For this review, take the finished solid that the model builds, in its own axes (mm). A direction names the side the tool comes from. Give positions to 0.01 mm unless a question says otherwise; leave off trailing zeros. Write each loop counter-clockwise with the first axis right and the second up, starting at its lowest first coordinate (ties: lowest second). Pieces come first, ordered by that corner, then holes. Notation, with made-up numbers: (56, 16) -> (81, 16) arc R30 cw to (81, 54) -> close; hole circle Ø3 at (-32, 41). An arc over 180 degrees is marked (long way). Answer as CSV lines item,"result".
```python
from build123d import *

# Parameters (mm, degrees)
SKETCH1_R           = 1.5
BOSS_EXTRUDE1_DEPTH = 3


with BuildPart() as part:
    # Sketch1 → Boss-Extrude1 (new body)
    with BuildSketch(Plane.XY):
        with BuildLine():
            ThreePointArc((-0.08, 4), (-0.080376511, 3.999992452), (-0.080753021, 3.999984869))
            ThreePointArc((-0.080753021, 3.999984869), (0.560266414, 4.536513248), (1.110799577, 5.165545722))
            Line((1.110799577, 5.165545722), (0.873535849, 5.738351032))
            ThreePointArc((0.873535849, 5.738351032), (-0.292204471, 5.779997685), (-1.43969018, 5.570327744))
            ThreePointArc((-1.43969018, 5.570327744), (-1.699752868, 6.045), (-1.980799756, 6.507557022))
            ThreePointArc((-1.980799756, 6.507557022), (-1.225477407, 7.396473826), (-0.678674306, 8.426857884))
            Line((-0.678674306, 8.426857884), (-1.056106392, 8.918736955))
            ThreePointArc((-1.056106392, 8.918736955), (-2.192904021, 8.657248736), (-3.247023529, 8.15773197))
            ThreePointArc((-3.247023529, 8.15773197), (-3.621079015, 8.548920985), (-4.01226803, 8.922976471))
            ThreePointArc((-4.01226803, 8.922976471), (-3.512751264, 9.977095979), (-3.251263045, 11.113893608))
            Line((-3.251263045, 11.113893608), (-3.743142116, 11.491325694))
            ThreePointArc((-3.743142116, 11.491325694), (-4.773526174, 10.944522593), (-5.662442978, 10.189200244))
            ThreePointArc((-5.662442978, 10.189200244), (-6.125, 10.470247132), (-6.599672256, 10.73030982))
            ThreePointArc((-6.599672256, 10.73030982), (-6.390002315, 11.877795529), (-6.431648968, 13.043535849))
            Line((-6.431648968, 13.043535849), (-7.004454278, 13.280799577))
            ThreePointArc((-7.004454278, 13.280799577), (-7.858205794, 12.485945322), (-8.521341684, 11.526291359))
            ThreePointArc((-8.521341684, 11.526291359), (-9.040877745, 11.67804324), (-9.566685112, 11.806390286))
            ThreePointArc((-9.566685112, 11.806390286), (-9.661150657, 12.969042942), (-10.003094031, 14.084282677))
            Line((-10.003094031, 14.084282677), (-10.617789845, 14.165208916))
            ThreePointArc((-10.617789845, 14.165208916), (-11.236727065, 13.176471511), (-11.628890424, 12.077884766))
            ThreePointArc((-11.628890424, 12.077884766), (-12.17, 12.09), (-12.711109576, 12.077884766))
            ThreePointArc((-12.711109576, 12.077884766), (-13.103272935, 13.176471511), (-13.722210155, 14.165208916))
            Line((-13.722210155, 14.165208916), (-14.336905969, 14.084282677))
            ThreePointArc((-14.336905969, 14.084282677), (-14.678849343, 12.969042942), (-14.773314888, 11.806390286))
            ThreePointArc((-14.773314888, 11.806390286), (-15.299122255, 11.67804324), (-15.818658316, 11.526291359))
            ThreePointArc((-15.818658316, 11.526291359), (-16.481794206, 12.485945322), (-17.335545722, 13.280799577))
            Line((-17.335545722, 13.280799577), (-17.908351032, 13.043535849))
            ThreePointArc((-17.908351032, 13.043535849), (-17.949997685, 11.877795529), (-17.740327744, 10.73030982))
            ThreePointArc((-17.740327744, 10.73030982), (-18.215, 10.470247132), (-18.677557022, 10.189200244))
            ThreePointArc((-18.677557022, 10.189200244), (-19.566473826, 10.944522593), (-20.596857884, 11.491325694))
            Line((-20.596857884, 11.491325694), (-21.088736955, 11.113893608))
            ThreePointArc((-21.088736955, 11.113893608), (-20.827248736, 9.977095979), (-20.32773197, 8.922976471))
            ThreePointArc((-20.32773197, 8.922976471), (-20.718920985, 8.548920985), (-21.092976471, 8.15773197))
            ThreePointArc((-21.092976471, 8.15773197), (-22.147095979, 8.657248736), (-23.283893608, 8.918736955))
            Line((-23.283893608, 8.918736955), (-23.661325694, 8.426857884))
            ThreePointArc((-23.661325694, 8.426857884), (-23.114522593, 7.396473826), (-22.359200244, 6.507557022))
            ThreePointArc((-22.359200244, 6.507557022), (-22.640247132, 6.045), (-22.90030982, 5.570327744))
            ThreePointArc((-22.90030982, 5.570327744), (-24.047795529, 5.779997685), (-25.213535849, 5.738351032))
            Line((-25.213535849, 5.738351032), (-25.450799577, 5.165545722))
            ThreePointArc((-25.450799577, 5.165545722), (-24.655945322, 4.311794206), (-23.696291359, 3.648658316))
            ThreePointArc((-23.696291359, 3.648658316), (-23.84804324, 3.129122255), (-23.976390286, 2.603314888))
            ThreePointArc((-23.976390286, 2.603314888), (-25.139042942, 2.508849343), (-26.254282677, 2.166905969))
            Line((-26.254282677, 2.166905969), (-26.335208916, 1.552210155))
            ThreePointArc((-26.335208916, 1.552210155), (-25.346471511, 0.933272935), (-24.247884766, 0.541109576))
            ThreePointArc((-24.247884766, 0.541109576), (-24.26, 0), (-24.247884766, -0.541109576))
            ThreePointArc((-24.247884766, -0.541109576), (-25.346471511, -0.933272935), (-26.335208916, -1.552210155))
            Line((-26.335208916, -1.552210155), (-26.254282677, -2.166905969))
            ThreePointArc((-26.254282677, -2.166905969), (-25.139042942, -2.508849343), (-23.976390286, -2.603314888))
            ThreePointArc((-23.976390286, -2.603314888), (-23.84804324, -3.129122255), (-23.696291359, -3.648658316))
            ThreePointArc((-23.696291359, -3.648658316), (-24.655945322, -4.311794206), (-25.450799577, -5.165545722))
            Line((-25.450799577, -5.165545722), (-25.213535849, -5.738351032))
            ThreePointArc((-25.213535849, -5.738351032), (-24.047795529, -5.779997685), (-22.90030982, -5.570327744))
            ThreePointArc((-22.90030982, -5.570327744), (-22.640247132, -6.045), (-22.359200244, -6.507557022))
            ThreePointArc((-22.359200244, -6.507557022), (-23.114522593, -7.396473826), (-23.661325694, -8.426857884))
            Line((-23.661325694, -8.426857884), (-23.283893608, -8.918736955))
            ThreePointArc((-23.283893608, -8.918736955), (-22.147095979, -8.657248736), (-21.092976471, -8.15773197))
            ThreePointArc((-21.092976471, -8.15773197), (-20.718920985, -8.548920985), (-20.32773197, -8.922976471))
            ThreePointArc((-20.32773197, -8.922976471), (-20.827248736, -9.977095979), (-21.088736955, -11.113893608))
            Line((-21.088736955, -11.113893608), (-20.596857884, -11.491325694))
            ThreePointArc((-20.596857884, -11.491325694), (-19.566473826, -10.944522593), (-18.677557022, -10.189200244))
            ThreePointArc((-18.677557022, -10.189200244), (-18.215, -10.470247132), (-17.740327744, -10.73030982))
            ThreePointArc((-17.740327744, -10.73030982), (-17.949997685, -11.877795529), (-17.908351032, -13.043535849))
            Line((-17.908351032, -13.043535849), (-17.335545722, -13.280799577))
            ThreePointArc((-17.335545722, -13.280799577), (-16.481794206, -12.485945322), (-15.818658316, -11.526291359))
            ThreePointArc((-15.818658316, -11.526291359), (-15.299122255, -11.67804324), (-14.773314888, -11.806390286))
            ThreePointArc((-14.773314888, -11.806390286), (-14.678849343, -12.969042942), (-14.336905969, -14.084282677))
            Line((-14.336905969, -14.084282677), (-13.722210155, -14.165208916))
            ThreePointArc((-13.722210155, -14.165208916), (-13.103272935, -13.176471511), (-12.711109576, -12.077884766))
            ThreePointArc((-12.711109576, -12.077884766), (-12.17, -12.09), (-11.628890424, -12.077884766))
            ThreePointArc((-11.628890424, -12.077884766), (-11.236727065, -13.176471511), (-10.617789845, -14.165208916))
            Line((-10.617789845, -14.165208916), (-10.003094031, -14.084282677))
            ThreePointArc((-10.003094031, -14.084282677), (-9.661150657, -12.969042942), (-9.566685112, -11.806390286))
            ThreePointArc((-9.566685112, -11.806390286), (-9.040877745, -11.67804324), (-8.521341684, -11.526291359))
            ThreePointArc((-8.521341684, -11.526291359), (-7.858205794, -12.485945322), (-7.004454278, -13.280799577))
            Line((-7.004454278, -13.280799577), (-6.431648968, -13.043535849))
            ThreePointArc((-6.431648968, -13.043535849), (-6.390002315, -11.877795529), (-6.599672256, -10.73030982))
            ThreePointArc((-6.599672256, -10.73030982), (-6.125, -10.470247132), (-5.662442978, -10.189200244))
            ThreePointArc((-5.662442978, -10.189200244), (-4.773526174, -10.944522593), (-3.743142116, -11.491325694))
            Line((-3.743142116, -11.491325694), (-3.251263045, -11.113893608))
            ThreePointArc((-3.251263045, -11.113893608), (-3.512751264, -9.977095979), (-4.01226803, -8.922976471))
            ThreePointArc((-4.01226803, -8.922976471), (-3.621079015, -8.548920985), (-3.247023529, -8.15773197))
            ThreePointArc((-3.247023529, -8.15773197), (-2.192904021, -8.657248736), (-1.056106392, -8.918736955))
            Line((-1.056106392, -8.918736955), (-0.678674306, -8.426857884))
            ThreePointArc((-0.678674306, -8.426857884), (-1.225477407, -7.396473826), (-1.980799756, -6.507557022))
            ThreePointArc((-1.980799756, -6.507557022), (-1.699752868, -6.045), (-1.43969018, -5.570327744))
            ThreePointArc((-1.43969018, -5.570327744), (-0.292204471, -5.779997685), (0.873535849, -5.738351032))
            Line((0.873535849, -5.738351032), (1.110799577, -5.165545722))
            ThreePointArc((1.110799577, -5.165545722), (0.560266414, -4.536513248), (-0.080753021, -3.999984869))
            ThreePointArc((-0.080753021, -3.999984869), (-0.080376511, -3.999992452), (-0.08, -4))
            Line((-0.08, -4), (18.91, -4))
            ThreePointArc((18.91, -4), (22.91, 0), (18.91, 4))
            Line((18.91, 4), (-0.08, 4))
        make_face()
        with Locations((18.91, 0)):
            Circle(SKETCH1_R, mode=Mode.SUBTRACT)
        with Locations((-12.17, 0)):
            Circle(SKETCH1_R, mode=Mode.SUBTRACT)
    extrude(amount=BOSS_EXTRUDE1_DEPTH)


solid = part.part
```
Q1. For faces 1 (the cylindrical face through (-25.332, -0.926, 1.479)), 2 (the cylindrical face through (-1.235, 7.383, 1.479)), 3 (the cylindrical face through (-11.244, -13.162, 1.479)), 4 (the cylindrical face through (-6.39, 11.86, 1.48)), list the 3-axis set-ups (+Z, -Z, +X, -X, +Y, -Y) from which the entire face can be reached by the end or side of a thin tool; tool diameter is ignored.
Answer block:
face 1,"+Z, -Z, -X"
face 2,"+Z, -Z, +X"
face 3,"+Z, -Z, -Y"
face 4,"+Z, -Z"
Q2. Add section B-B (y = 0). Write out the cut boundary in (x, z), plus the area to 3 significant figures.
Answer block:
outline,"(-24.26, 0) -> (-13.67, 0) -> (-13.67, 3) -> (-24.26, 3) -> close; (-10.67, 0) -> (17.41, 0) -> (17.41, 3) -> (-10.67, 3) -> close; (20.41, 0) -> (22.91, 0) -> (22.91, 3) -> (20.41, 3) -> close"
area,"124 mm2"
Q3. Draft analysis for pull direction X (two halves, no side actions). For faces 5 (the cylindrical face through (-23.124, 7.41, 1.479)), 6 (the cylindrical face through (-16.47, 12.47, 1.48)), 7 (the flat face through (-8, 0, 0)), state which applies: released by +X, released by -X, zero draft, split by the parting line, or undercut.
Answer block:
face 5,"released by -X"
face 6,"undercut"
face 7,"zero draft"
Q4. Add section A-A (x = -12.17). Write out the cut boundary in (y, z).
Answer block:
outline,"(-12.09, 0) -> (-1.5, 0) -> (-1.5, 3) -> (-12.09, 3) -> close; (1.5, 0) -> (12.09, 0) -> (12.09, 3) -> (1.5, 3) -> close"
Q5. Clearance check with a flat-ended pin moving along its axis: pin 1 (1.5 mm diameter, centred on x = -19.5, z = 2.5, fed in from -Y). State where the tip first meets the part, or that it passes through.
Answer block:
pin 1,"stops at y = -11.34"
Q6. Add section D-D (x = 10.5). Write out the cut boundary in (y, z), plus the area to 3 significant figures.
Answer block:
outline,"(-4, 0) -> (4, 0) -> (4, 3) -> (-4, 3) -> close"
area,"24.0 mm2"
Q7. To check wall thickness, follow probe 1 along Y at (x, z) = (-12.17, 2.2); probe 2 along Y at (x, z) = (18.91, 1); probe 3 along Y at (x, z) = (-23, 1.25). State the ranges of each line that lie inside material, in increasing order. Write a range as [from, to].
Answer block:
probe 1,"y = [-12.09, -1.5], [1.5, 12.09]"
probe 2,"y = [-4, -1.5], [1.5, 4]"
probe 3,"y = [-8.88, -7.23], [-5.6, 5.6], [7.23, 8.88]"
Q8. Add section C-C (z = 1.2). State how many separate pieces and enclosed holes the cut face has, plus the area to 3 significant figures.
Answer block:
separate pieces,"1"
enclosed holes,"2"
area,"696 mm2"
